```python
from build123d import *

# Parameters (mm, degrees)
SKETCH_R     = 1.6
PAD_DEPTH    = 3
PAD001_DEPTH = 20
SKETCH002_W  = 9.48
SKETCH002_H  = 9.48
POCKET_DEPTH = 1.56
CHAMFER_SIZE = 9
FILLET_R     = 3


with BuildPart() as part:
    # Sketch → Pad (new body)
    with BuildSketch(Plane.XY):
        Polygon((-10, 10), (10, 10), (10, -10), (-10, -10), (-20, -10), (-20, 10), align=None)
        Circle(SKETCH_R, mode=Mode.SUBTRACT)
        with BuildLine():
            ThreePointArc((-15.9, 1.6), (-17.5, 0), (-15.9, -1.6))
            Line((-15.9, -1.6), (-11.6, -1.6))
            ThreePointArc((-11.6, -1.6), (-10, 0), (-11.6, 1.6))
            Line((-11.6, 1.6), (-15.9, 1.6))
        make_face(mode=Mode.SUBTRACT)
    extrude(amount=PAD_DEPTH)

    # Sketch001 (on Face3 of Pad) → Pad001 (join)
    with BuildSketch(Plane.XZ.offset(10)):
        Polygon((-4.74, 3), (4.74, 3), (2.94, 4.56), (-2.94, 4.56), align=None)
    extrude(amount=-PAD001_DEPTH)

    # Sketch002 (on Face18 of Pad001) → Pocket (cut)
    with BuildSketch(Plane.XY.offset(4.56)):
        Rectangle(SKETCH002_W, SKETCH002_H)
    extrude(amount=-POCKET_DEPTH, mode=Mode.SUBTRACT)

    # Chamfer
    chamfer_edges = [part.edges().sort_by_distance(p)[0] for p in [
        (-20, 10, 1.5),
        (-20, -10, 1.5),
    ]]
    chamfer(chamfer_edges, length=CHAMFER_SIZE)

    # Fillet
    fillet_edges = [part.edges().sort_by_distance(p)[0] for p in [
        (10, -10, 1.5),
        (10, 10, 1.5),
    ]]
    fillet(fillet_edges, radius=FILLET_R)


solid = part.part
```
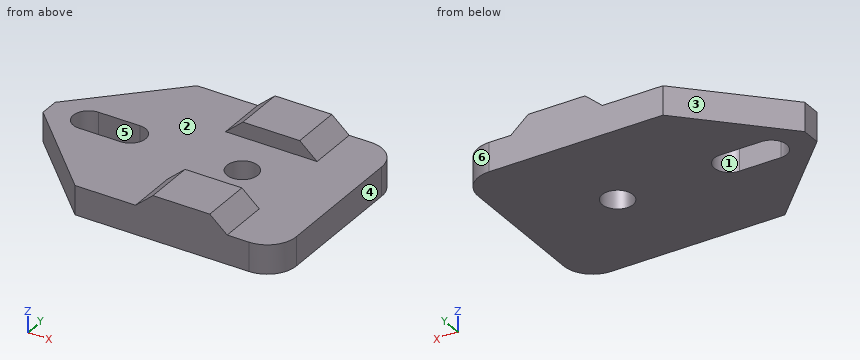
The model under review builds one solid part; all positions refer to its coordinate system, in mm. Face numbers are marked on the shaded views. A direction names the side the tool comes from. Round coordinates to 2 decimals unless told otherwise and drop trailing zeros. Write each loop counter-clockwise with the first axis right and the second up, starting at its lowest first coordinate (ties: lowest second). Pieces come first, ordered by that corner, then holes.
(1) We need section C-C on z = 3.95. Give the boundary of the cut face in (x, y), and give its area (3 significant figures).
(2) We need section A-A on x = 0. Give the boundary of the cut face in (y, z), and give its area (3 significant figures).
(3) Wall thickness on L1, parallel to Y at x = 0, z = 0.95; L2, parallel to Z at x = -13.25, y = -7; L3, parallel to Y at x = -2.25, z = 3.7: over which ranges is each line inside the solid? List them lowest first.
(4) Mouldability with a two-part tool opening along Y and no side actions: class the marked faces 4, 5 and 6 as +Y half, -Y half, draft (parallel to the pull), parting line (faces both ways), or undercut.
(5) We need section D-D on y = 2.5. Give the boundary of the cut face in (x, z), and give its area (3 significant figures).
(6) Insertion check: pin 1 (0.9 mm diameter, centred on x = -13, z = 2, fed in from -Y); pin 2 (2.5 mm diameter, centred on x = 0, y = 0, fed in from -Z); pin 3 (1.5 mm diameter, centred on x = -14.5, z = 2, fed in from +Y). Each pin has a flat end and moves straight along its axis. Give the tip position at first contact, or say it passes through.
(7) Machinability: for the marked faces 1, 2 and 3, which of the approach directions +Z, -Z, +X, -X, +Y, -Y give a long, thin tool a straight path to every point of the face, cutting with its end or side? Answer none if there is none.
(8) We need section B-B on y = 0. Give the boundary of the cut face in (x, z).
Findings below:
1. outline: (-3.64, -10) - (3.64, -10) - (3.64, -4.74) - (-3.64, -4.74) - close; (-3.64, 4.74) - (3.64, 4.74) - (3.64, 10) - (-3.64, 10) - close
1. area: 76.7 mm2
2. outline: (-10, 0) - (-1.6, 0) - (-1.6, 3) - (-4.74, 3) - (-4.74, 4.56) - (-10, 4.56) - close; (1.6, 0) - (10, 0) - (10, 4.56) - (4.74, 4.56) - (4.74, 3) - (1.6, 3) - close
2. area: 66.8 mm2
3. L1: y = -10 to -1.6, 1.6 to 10
3. L2: z = 0 to 3
3. L3: y = -10 to -4.74, 4.74 to 10
4. face 4: draft
4. face 5: undercut
4. face 6: +Y half
5. outline: (-18.5, 0) - (10, 0) - (10, 3) - (-18.5, 3) - close
5. area: 85.5 mm2
6. pin 1: stops at y = -8.45
6. pin 2: passes through
6. pin 3: stops at y = 7.25
7. face 1: +Z, -Z
7. face 2: +Z
7. face 3: +Z, -Z, -X, +Y
8. outline: (-20, 0) - (-17.5, 0) - (-17.5, 3) - (-20, 3) - close; (-10, 0) - (-1.6, 0) - (-1.6, 3) - (-10, 3) - close; (1.6, 0) - (10, 0) - (10, 3) - (1.6, 3) - close
